Input: part model. Units: mm. Frame: model coordinates. A direction names the side the tool comes from. Round coordinates to 2 decimals unless told otherwise and drop trailing zeros. Loops run counter-clockwise (first coordinate to the right, second up) from the corner with the lowest first, then second, coordinate; pieces in that order, holes last. Notation, with made-up numbers: (80, -15.75) - (115, -15.75) arc R31 ccw to (115, 20.25) - close; hole circle Ø10 at (77.25, -5.5). An arc over 180 degrees is marked (long way). One line per question, with ' | ' between items. Start each with the question number.
Item 1: Set-up query: faces 1 (the face through (169.7, -6.2, 53.182)), 2 (the face through (157.535, -12, 62)), 3 (the face through (-3, -37, 5)), 4 (the face through (197.465, -13, 63)), 5 (the face through (0, 14, -20)). Return all of +Z, -Z, +X, -X, +Y, -Y with unobstructed straight access to the full face (end or side cutting, diameter ignored); none if empty.
Item 2: Section B-B, the plane x = 138. Return loops of the section in (y, z), plus the area to 3 significant figures.
Item 3: First-contact query: pin 1 (10 mm diameter, centred on x = 152, y = 11, fed in from -Z); pin 2 (7 mm diameter, centred on y = -7, z = 61, fed in from +X) (3 decimals); pin 3 (10 mm diameter, centred on x = 194, z = 55.5, fed in from -Y). Flat tips, straight axial feed; report the tip coordinate or a pass-through.
Item 4: Section C-C, the plane z = 18. Return loops of the section in (x, y) (1 decimal), plus the area to 3 significant figures.
Item 5: Section D-D, the plane y = -34.5. Return loops of the section in (x, z).
Item 6: Material intervals for line 1 along Y through (x, z) = (175, 56) (1 decimal); line 2 along Z through (x, y) = (-50.5, -34.5); line 3 along Y through (x, z) = (-175, 69.3) (1 decimal), sorted ascending.
Item 7: Section A-A, the plane y = -16. Return loops of the section in (x, z) (3 decimals).
Item 8: Draft query along Z for faces 6 (the face through (-4, -40, 71.818)), 7 (the face through (175, -25, 57)), 8 (the face through (-152.535, -13, 63)). Return one class per face: pulls with the +Z half, pulls with the -Z half, needs draft (parallel to the pull), parting line crosses it, or undercut.
```python
from build123d import *

# Parameters (mm, degrees)
BOSS_EXTRUDE7_DEPTH = 71.818
SHELL8_START        = 5
SHELL8_DEPTH        = 61.818
BOSS_EXTRUDE4_DEPTH = 18.636
SHELL7_START        = 58.182
SHELL7_DEPTH        = 8.636
SKETCH5_R           = 7.9375
CUT_EXTRUDE1_DEPTH  = 274.461475598
BOSS_EXTRUDE5_DEPTH = 5
BOSS_EXTRUDE6_DEPTH = 20


# Read off the part's stored shape, not the designer's step: Shell8, Shell7
with BuildPart() as part:
    # Sketch3 → Boss-Extrude7 (new body)
    with BuildSketch(Plane.XY):
        with BuildLine():
            ThreePointArc((-251.338111427, -25), (-222.139790815, -65.041120671), (-175, -80.3275))
            Line((-175, -80.3275), (175, -80.3275))
            ThreePointArc((175, -80.3275), (222.139790815, -65.041120671), (251.338111427, -25))
            Line((251.338111427, -25), (-251.338111427, -25))
        make_face()
    extrude(amount=BOSS_EXTRUDE7_DEPTH)

    # Shell8 outline → Shell8 (cut)
    with BuildSketch(Plane.XY.offset(SHELL8_START)):
        with BuildLine():
            ThreePointArc((-246.057949986, -25), (-218.537597294, -61.471211783), (-175, -75.3275))
            Line((-175, -75.3275), (175, -75.3275))
            ThreePointArc((175, -75.3275), (218.537597294, -61.471211783), (246.057949986, -25))
            Line((246.057949986, -25), (-246.057949986, -25))
        make_face()
    extrude(amount=SHELL8_DEPTH, mode=Mode.SUBTRACT)

    # Sketch4 → Boss-Extrude4 (add)
    with BuildSketch(Plane.XY.offset(71.818)):
        with BuildLine():
            Line((152.535, -25), (197.465, -25))
            Line((197.465, -25), (197.465, 0))
            ThreePointArc((197.465, 0), (175, 22.465), (152.535, 0))
            Line((152.535, 0), (152.535, -25))
        make_face()
        with BuildLine():
            Line((-197.465, 0), (-197.465, -25))
            Line((-197.465, -25), (-152.535, -25))
            Line((-152.535, -25), (-152.535, 0))
            ThreePointArc((-152.535, 0), (-175, 22.465), (-197.465, 0))
        make_face()
    extrude(amount=-BOSS_EXTRUDE4_DEPTH)

    # Shell7 outline → Shell7 (cut)
    with BuildSketch(Plane.XY.offset(SHELL7_START)):
        with BuildLine():
            Line((192.465, -25), (192.465, 0))
            ThreePointArc((192.465, 0), (175, 17.465), (157.535, 0))
            Line((157.535, 0), (157.535, -25))
            Line((157.535, -25), (192.465, -25))
        make_face()
        with BuildLine():
            ThreePointArc((-157.535, 0), (-175, 17.465), (-192.465, 0))
            Line((-192.465, 0), (-192.465, -25))
            Line((-192.465, -25), (-157.535, -25))
            Line((-157.535, -25), (-157.535, 0))
        make_face()
    extrude(amount=SHELL7_DEPTH, mode=Mode.SUBTRACT)

    # Sketch5 → Cut-Extrude1 (cut, through all)
    with BuildSketch(Plane.XY.offset(71.818)):
        with Locations((175, 0)):
            Circle(SKETCH5_R)
        with Locations((-175, 0)):
            Circle(SKETCH5_R)
    extrude(amount=-CUT_EXTRUDE1_DEPTH, mode=Mode.SUBTRACT)

    # Sketch13 → Boss-Extrude5 (add)
    with BuildSketch(Plane(origin=(0, 0, 0), x_dir=(-1, 0, 0), z_dir=(0, 0, -1))):
        Polygon((131.634946049, -25), (132.910361442, 11.477741548), (-131.784153156, 20.732575975), (-133.383156517, -25), align=None)
    extrude(amount=-BOSS_EXTRUDE5_DEPTH)

    # Sketch14 → Boss-Extrude6 (add)
    with BuildSketch(Plane(origin=(0, 0, 0), x_dir=(-1, 0, 0), z_dir=(0, 0, -1))):
        Polygon((-131.784153156, 20.732575975), (-131.958867442, 15.735629415), (132.735647156, 6.480794988), (132.910361442, 11.477741548), align=None)
    extrude(amount=BOSS_EXTRUDE6_DEPTH)


solid = part.part
```
Return value:
1) face 1: -Z, +X, -X, +Y | face 2: none | face 3: +Y | face 4: +Z, -Z, +X, +Y | face 5: -Z, +X, -X, +Y, -Y
2) outline: (-80.33, 0) - (-25, 0) - (-25, 5) - (-75.33, 5) - (-75.33, 66.82) - (-25, 66.82) - (-25, 71.82) - (-80.33, 71.82) - close | area: 862 mm2
3) pin 1: z = 53.18 | pin 2: x = 197.465 | pin 3: y = -79.1
4) outline: (-251.3, -25) arc R80.3 ccw to (-175, -80.3) - (175, -80.3) arc R80.3 ccw to (251.3, -25) - (246.1, -25) arc R75.3 cw to (175, -75.3) - (-175, -75.3) arc R75.3 cw to (-246.1, -25) - close | area: 2,720 mm2
5) outline: (-247.54, 0) - (247.54, 0) - (247.54, 71.82) - (-247.54, 71.82) - close; hole (-241.96, 5) - (241.96, 5) - (241.96, 66.82) - (-241.96, 66.82) - close
6) line 1: -80.3 to -75.3, -25 to -7.9, 7.9 to 22.5 | line 2: 0 to 5, 66.82 to 71.82 | line 3: -80.3 to -7.9, 7.9 to 22.5
7) outline: (-197.465, 53.182) - (-152.535, 53.182) - (-152.535, 71.818) - (-197.465, 71.818) - close; (-131.95, 0) - (133.068, 0) - (133.068, 5) - (-131.95, 5) - close; (152.535, 53.182) - (197.465, 53.182) - (197.465, 71.818) - (152.535, 71.818) - close; hole (-192.465, 58.182) - (-157.535, 58.182) - (-157.535, 66.818) - (-192.465, 66.818) - close; hole (157.535, 58.182) - (192.465, 58.182) - (192.465, 66.818) - (157.535, 66.818) - close
8) face 6: pulls with the +Z half | face 7: undercut | face 8: needs draft
